```python
from build123d import *

# Parameters (mm, degrees)
BOSS_EXTRU_1_DEPTH      = 3
CONG_1_R                = 10
CONG_2_R                = 1
CONG_3_R                = 1
ESQUISSE2_R             = 1.25
ENL_V_MAT_EXTRU_1_DEPTH = 26.341724021


with BuildPart() as part:
    # Esquisse1 → Boss.-Extru.1 (new, symmetric)
    with BuildSketch(Plane(origin=(0, 0, 0), x_dir=(0, 0, -1), z_dir=(1, 0, 0))):
        with BuildLine():
            Line((0, 0), (0, 10))
            Line((0, 10), (-8, 10))
            Line((-8, 10), (-8, 16.390227771))
            ThreePointArc((-8, 16.390227771), (-9.505336244, 17.8453296), (-10.357829377, 19.757557096))
            Line((-10.357829377, 19.757557096), (-20.121449742, 23.311224288))
            Line((-20.121449742, 23.311224288), (-21.489530315, 19.552453804))
            Line((-21.489530315, 19.552453804), (-20, 0))
            Line((-20, 0), (0, 0))
        make_face()
    extrude(amount=BOSS_EXTRU_1_DEPTH, both=True)

    # Congé1
    cong_1_edges = [part.edges().sort_by_distance(p)[0] for p in [
        (0, 19.552453804, 21.489530315),
    ]]
    fillet(cong_1_edges, radius=CONG_1_R)

    # Congé2
    cong_2_edges = [part.edges().sort_by_distance(p)[0] for p in [
        (0, 10, 8),
    ]]
    fillet(cong_2_edges, radius=CONG_2_R)

    # Congé3
    cong_3_edges = [part.edges().sort_by_distance(p)[0] for p in [
        (-3, 10, 3.5),
        (3, 21.534390692, 15.239639559),
        (3, 22.445813748, 20.436433419),
        (-3, 8.700295175, 20.662799337),
        (3, 8.700295175, 20.662799337),
        (-3, 19.521122757, 21.261452787),
        (3, 19.521122757, 21.261452787),
        (-3, 13.695113886, 8),
        (3, 13.695113886, 8),
        (-3, 10.292893219, 7.707106781),
        (3, 10.292893219, 7.707106781),
        (3, 10, 3.5),
        (-3, 22.445813748, 20.436433419),
        (-3, 21.534390692, 15.239639559),
    ]]
    fillet(cong_3_edges, radius=CONG_3_R)

    # Esquisse2 → Enlèv. mat.-Extru.1 (cut, through all)
    with BuildSketch(Plane(origin=(0, 10, 0), x_dir=(1, 0, 0), z_dir=(0, 1, 0))):
        with Locations(Location((0, -5, 0), (0, 0, 270))):
            Circle(ESQUISSE2_R)
    extrude(amount=-ENL_V_MAT_EXTRU_1_DEPTH, mode=Mode.SUBTRACT)


solid = part.part
```
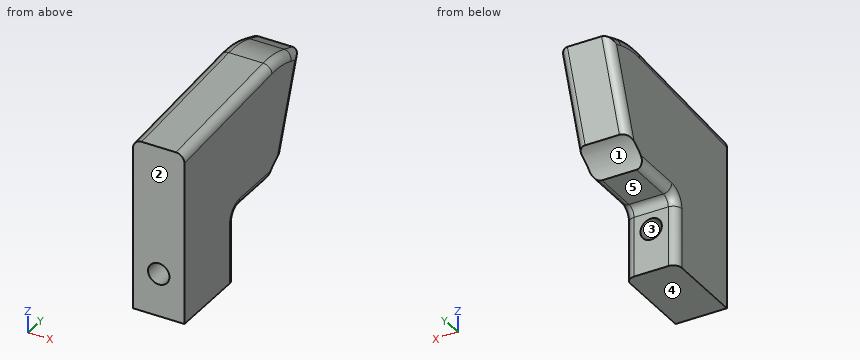
Geometry check sheet. Reference: the model listing, model coordinates, mm. Face numbers are marked on the shaded views. A direction names the side the tool comes from. Give positions to 0.01 mm unless a question says otherwise; leave off trailing zeros. Order: outer loops, then holes, each group sorted by start corner. A loop starts at its lowest first (then second) coordinate and runs counter-clockwise, first axis right, second up.
1. Release check for a two-part mould opening along Z. For the marked faces 1, 2 and 3 record: pulls with the +Z half, pulls with the -Z half, needs draft (parallel to the pull), parting line crosses it, or undercut.
2. Access from +Z, -Z, +X, -X, +Y, -Y to the whole of each face (thin tool, end or side, straight path). Record for the marked faces 4 and 5.
3. Section check B-B, the plane z = 5. Enter the section's corners in (x, y).
4. Section check A-A, the plane x = 0. Enter the section's corners in (y, z).
5. Gauge pin test, flat ends, axial feed: pin 1 Ø3 at (x, y) = (1, 7.5) entering from +Z; pin 2 Ø1.2 at (x, y) = (1, 12.5) entering from -Z; pin 3 Ø1 at (x, z) = (-1, 17.5) entering from +Y. Record the tip position at first contact, or that the pin passes through.
6. Thickness scan on L1, parallel to X at y = 4, z = 5; L2, parallel to Y at x = -2.25, z = 7.25; L3, parallel to Z at x = -1, y = 7. Record the ranges inside material, lowest first.
Values follow:
1. face 1: pulls with the -Z half
1. face 2: needs draft
1. face 3: undercut
2. face 4: -Z, +X, -X, +Y, -Y
2. face 5: -Z, +X, -X, +Y
3. outline: (-3, 0) - (-1.25, 0) - (-1.25, 10) - (-2, 10) arc R1 ccw to (-3, 9) - close; (1.25, 0) - (3, 0) - (3, 9) arc R1 ccw to (2, 10) - (1.25, 10) - close
4. outline: (0, 0) - (10, 0) - (10, 3.75) - (0, 3.75) - close; (0, 6.25) - (10, 6.25) - (10, 7) arc R1 cw to (11, 8) - (16.39, 8) arc R5.5 cw to (19.76, 10.36) - (23.31, 20.12) - (21.58, 20.75) arc R10 ccw to (17.4, 21.33) - (0, 20) - close
5. pin 1: stops at z = 20.69
5. pin 2: stops at z = 8
5. pin 3: stops at y = 22.54
6. L1: x = -3 to -1.25, 1.25 to 3
6. L2: y = 0 to 10
6. L3: z = 0 to 4.25, 5.75 to 20.53
